Autodesk Fusion 360 part; units mm, degrees
sketch "Sketch1" plane through (0, 22, 0) normal (0, 1, 0) x (-1, 0, 0)
  line L0 (11.5698, 0.25) -> (15.3, 0.25)
  line L1 (15.3, 0.25) -> (15.3, -0.5)
  line L2 (15.3, -0.5) -> (15.6004, -0.5)
  line L3 (15.6004, -0.5) -> (15.6004, -1.2)
  line L4 (15.6004, -1.2) -> (16.0004, -1.2)
  line L5 (16.0004, -1.2) -> (16.0004, -0.5)
  line L6 (16.0004, -0.5) -> (16.3, -0.5)
  line L7 (16.3, -0.5) -> (16.3, 1.05)
  line L8 (16.3, 1.05) -> (5, 1.05)
  line L9 (11.5698, -1.2) -> (11.5698, 0.25)
  line L10 (11.5698, -0.6208) -> (11.2698, -0.6208) construction
  line L11 (11.2698, -0.5) -> (11.2698, -1.2)
  line L12 (11.2698, -0.5) -> (10.5698, -0.5)
  line L13 (10.5698, -0.5) -> (10.5698, -1.2)
  line L14 (10.5698, -0.678) -> (10.2698, -0.678) construction
  line L15 (10.2698, 1.05) -> (10.2698, -1.2)
  line L16 (10.2698, 1.05) -> (16.3, 1.05)
  line L17 (16.3, -0.5) -> (16.0004, -0.5)
  line L18 (16.0004, -1.2) -> (15.6004, -1.2)
  line L19 (15.6004, -0.5) -> (15.3, -0.5)
  line L20 (15.3, 0.25) -> (11.5698, 0.25)
  line L21 (11.5698, -1.2) -> (11.2698, -1.2)
  line L22 (11.5698, -1.2) -> (11.2698, -1.2)
  line L23 (11.2698, -0.5) -> (10.5698, -0.5)
  line L24 (10.5698, -1.2) -> (10.2698, -1.2)
  line L25 (10.2698, 1.05) -> (16.3, 1.05)
  line L26 (16.3, -0.5) -> (16.0004, -0.5)
  line L27 (16.0004, -1.2) -> (15.6004, -1.2)
  line L28 (15.6004, -0.5) -> (15.3, -0.5)
  line L29 (15.3, 0.25) -> (11.5698, 0.25)
  dimension "d14" = 0.3
  dimension "d15" = 0.7
  dimension "d16" = 0.3
extrude "Extrude1" add sketch "Sketch1" along normal blind 8.2 makes body 1
copy_body "Body->Comp1" bodies 1 removing the originals makes body 2 in component "Component"
move_face "OffsetFaces1" offset 0.3 1 faces at (-12.8132, 24.7333, 0.25) on bodies 2 in component "Component"
move_face "OffsetFaces2" offset -0.4 1 faces at (-12.2798, 27.4667, 1.05) on bodies 2 in component "Component"
move_face "OffsetFaces3" offset 3.3 1 faces at (-10.2698, 24.7333, 0.0333) on bodies 2 in component "Component"
move_face "OffsetFaces4" offset -3.3 1 faces at (-10.5698, 24.7333, -0.7333) on bodies 2 in component "Component"
move_face "OffsetFaces5" offset 3.3 1 faces at (-11.2698, 24.7333, -0.7333) on bodies 2 in component "Component"
move_face "OffsetFaces6" offset -3.3 1 faces at (-11.5698, 27.4667, -0.8167) on bodies 2 in component "Component"
move_face "OffsetFaces7" offset -4.2 1 faces at (-10.5132, 22, 0.4167) on bodies 2 in component "Component"
move_face "OffsetFaces8" offset -0.1 1 faces at (-8.2698, 28.8667, -0.4333) on bodies 2 in component "Component"
move_face "OffsetFaces9" offset 0.1 1 faces at (-7.9698, 27.5333, -0.7333) on bodies 2 in component "Component"
component "Component" placed x (1, 0, 0) y (0, 1, 0) z (0, 0, 1) at (0, 0, 0)
Read the model definition and answer for the solid it produces. Units are mm, in the model's axes. A direction names the side the tool comes from. Give positions to 0.01 mm unless a question says otherwise; leave off trailing zeros. Write each loop counter-clockwise with the first axis right and the second up, starting at its lowest first coordinate (ties: lowest second). Pieces come first, ordered by that corner, then holes. Notation, with made-up numbers: (89, -25.75) - (141, -25.75) arc R24 cw to (141, -9.75) - close; hole circle Ø11 at (80.25, 42.5). An arc over 180 degrees is marked (long way). Return JSON: item names as keys, results as strings.
Q1. Given P1, Ø1.2, axis at x = -13, y = 28, coming from the -Z side, flat-ended and moving along its own axis, determine where the tip first touches the part or whether it passes through.
Reply:
{"P1": "z = -0.05"}
Q2. A cutting plane is placed at D-D, the plane x = -13. Determine the outline of the cut face in (y, z), and give its area (3 significant figures).
Reply:
{"outline": "(26.2, -0.05) - (30.2, -0.05) - (30.2, 0.65) - (26.2, 0.65) - close", "area": "2.80 mm²"}
Q3. Consider line 1 along X through (y, z) = (28.5, -0.9); line 2 along X through (y, z) = (27.3, -0.45); line 3 along Z through (x, y) = (-13.5, 26.6). Determine where each line is inside the solid, lowest interval first. Write a range as [from, to].
Reply:
{"line 1": "[-16, -15.6], [-8.17, -7.87], [-7.27, -6.97]", "line 2": "[-16.3, -15.3], [-8.17, -6.97]", "line 3": "[-0.05, 0.65]"}
Q4. For a pull along Y with two mould halves and no side action, classify faces 3 (the face through (-12, 28, 0.65)), 4 (the face through (-11.6, 26.2, 0.1)), 5 (the face through (-11.6, 30.2, 0.1)) as released by +Y, released by -Y, zero draft, split by the parting line, or undercut.
Reply:
{"face 3": "zero draft", "face 4": "released by -Y", "face 5": "released by +Y"}
Q5. A cutting plane is placed at A-A, the plane z = -0.3. Determine the outline of the cut face in (x, y), and give its area (3 significant figures).
Reply:
{"outline": "(-16.3, 26.2) - (-15.3, 26.2) - (-15.3, 30.2) - (-16.3, 30.2) - close; (-8.17, 26.2) - (-6.97, 26.2) - (-6.97, 30.2) - (-8.17, 30.2) - close", "area": "8.80 mm²"}
Q6. For faces 1 (the face through (-8.17, 28, -1)), 2 (the face through (-16.3, 28, 0)), determine the directions among +Z, -Z, +X, -X, +Y, -Y from which every point of the face is accessible in a straight line to the end or side of a thin tool.
Reply:
{"face 1": "-Z, +Y, -Y", "face 2": "+Z, -Z, -X, +Y, -Y"}
Q7. A cutting plane is placed at C-C, the plane y = 27.2. Determine the outline of the cut face in (x, z).
Reply:
{"outline": "(-16.3, -0.5) - (-16, -0.5) - (-16, -1.2) - (-15.6, -1.2) - (-15.6, -0.5) - (-15.3, -0.5) - (-15.3, -0.05) - (-8.17, -0.05) - (-8.17, -1.2) - (-7.87, -1.2) - (-7.87, -0.5) - (-7.27, -0.5) - (-7.27, -1.2) - (-6.97, -1.2) - (-6.97, 0.65) - (-16.3, 0.65) - close"}
Q8. A cutting plane is placed at B-B, the plane z = -0.75. Determine the outline of the cut face in (x, y), and give its area (3 significant figures).
Reply:
{"outline": "(-16, 26.2) - (-15.6, 26.2) - (-15.6, 30.2) - (-16, 30.2) - close; (-8.17, 26.2) - (-7.87, 26.2) - (-7.87, 30.2) - (-8.17, 30.2) - close; (-7.27, 26.2) - (-6.97, 26.2) - (-6.97, 30.2) - (-7.27, 30.2) - close", "area": "4.00 mm²"}
